```python
from build123d import *

# Parameters (mm, degrees)
SKETCH1_W           = 15.9
SKETCH1_H           = 7.95
BOSS_EXTRUDE1_DEPTH = 3.2
SHELL1_T            = -1.2
SKETCH3_R           = 1.525
SKETCH3_R_2         = 0.5
BOSS_EXTRUDE3_DEPTH = 2
BOSS_EXTRUDE4_DEPTH = 9
SKETCH7_W           = 30
SKETCH7_H           = 30
CUT_EXTRUDE1_DEPTH  = 14.969416324
BOSS_EXTRUDE5_START = -5.621499
SKETCH8_R           = 1.35
BOSS_EXTRUDE5_DEPTH = 5.621499


with BuildPart() as part:
    # Sketch1 → Boss-Extrude1 (new body)
    with BuildSketch(Plane(origin=(0, 0, 0), x_dir=(1, 0, 0), z_dir=(0, 1, 0))):
        Rectangle(SKETCH1_W, SKETCH1_H)
    extrude(amount=BOSS_EXTRUDE1_DEPTH)

    # Shell1
    shell1_openings = [part.faces().sort_by_distance(p)[0] for p in [
        (0, 0, 0),
    ]]
    offset(amount=SHELL1_T, openings=shell1_openings, kind=Kind.INTERSECTION)

    # Sketch3 → Boss-Extrude3 (add)
    with BuildSketch(Plane.XZ.offset(-2)):
        with Locations(Location((0, 0, 0), (0, 0, 270))):
            Circle(SKETCH3_R)
        with Locations(Location((0, 0, 0), (0, 0, 270))):
            Circle(SKETCH3_R_2, mode=Mode.SUBTRACT)
    extrude(amount=BOSS_EXTRUDE3_DEPTH)

    # Sketch4 → Boss-Extrude4 (add)
    with BuildSketch(Plane(origin=(0, 3.2, 0), x_dir=(1, 0, 0), z_dir=(0, 1, 0))):
        with BuildLine():
            Line((-3.9, 3.975), (-3.9, 2.475))
            Line((-3.9, 2.475), (-2.598076211, 2.475))
            ThreePointArc((-2.598076211, 2.475), (0, 0.975), (2.598076211, 2.475))
            Line((2.598076211, 2.475), (3.9, 2.475))
            Line((3.9, 2.475), (3.9, 3.975))
            Line((3.9, 3.975), (-3.9, 3.975))
        make_face()
    extrude(amount=BOSS_EXTRUDE4_DEPTH)

    # Sketch7 → Cut-Extrude1 (cut, through all)
    with BuildSketch(Plane(origin=(0, 4.863093078, 4.863093078), x_dir=(1, 0, 0), z_dir=(0, 0.7071067811865475, 0.7071067811865477))):
        Rectangle(SKETCH7_W, SKETCH7_H)
    extrude(amount=CUT_EXTRUDE1_DEPTH, mode=Mode.SUBTRACT)

    # Sketch8 → Boss-Extrude5 (add)
    with BuildSketch(Plane(origin=(0, 8.0875, 8.0875), x_dir=(1, 0, 0), z_dir=(0, 0.7071067811865475, 0.7071067811865477)).offset(BOSS_EXTRUDE5_START)):
        with Locations(Location((0, 10.087452186, 0), (0, 0, 270))):
            Circle(SKETCH8_R)
    extrude(amount=BOSS_EXTRUDE5_DEPTH)


solid = part.part
```
Build history of the part. All positions in model axes, mm. A direction names the side the tool comes from. Round coordinates to 2 decimals unless told otherwise and drop trailing zeros. Write each loop counter-clockwise with the first axis right and the second up, starting at its lowest first coordinate (ties: lowest second). Pieces come first, ordered by that corner, then holes. Notation, with made-up numbers: (-9, -20.5) - (17, -20.5) arc R22 ccw to (17, 4.5) - close; hole circle Ø9 at (40.5, -8.5). An arc over 180 degrees is marked (long way). Write each question's results on one line, items separated by ' | '. Start each with the question number.
Item 1: Mould opens along Z. For faces 5 (the face through (0, 2, 3.975)), 6 (the face through (3.9, 8, -3)), 7 (the face through (-6.75, 1, 0)) say: pulls with the +Z half, pulls with the -Z half, needs draft (parallel to the pull), parting line crosses it, or undercut.
Item 2: Wall check: L1, parallel to X at y = 0.75, z = 0 (3 decimals); L2, parallel to Z at x = -6.25, y = 1.75 (3 decimals); L3, parallel to Y at x = 4.75, z = 1. Give the ranges that are in metal, low to high. Write a range as [from, to].
Item 3: Saw through at B-B (y = 5.5). Write the cut outline in (x, z) (3 decimals).
Item 4: Saw through at C-C (x = 2.25). Write the cut outline in (y, z) (3 decimals), and give its area (3 significant figures).
Item 5: Saw through at D-D (x = -0.75). Write the cut outline in (y, z) (3 decimals), and give its area (3 significant figures).
Item 6: Saw through at A-A (x = -5.75). Write the cut outline in (y, z) (3 decimals).
Item 7: Which spindle directions (+Z, -Z, +X, -X, +Y, -Y) get a long thin tool onto all of the face, cutting with end or side? Do faces 1 (the face through (3, 8, -2.475)), 2 (the face through (0, 5, -3.975)), 3 (the face through (-0.93, 1.01, 1.21)), 4 (the face through (-3.9, 8, -3)). Say none if no direction does.
Item 8: Drop flat-ended pins along their axis: P1, Ø1.7, axis at x = -3, z = -3, coming from the +Y side; P2, Ø4, axis at x = -6.5, y = 3.5, coming from the +Z side (3 decimals); P3, Ø1.2, axis at x = 1.5, z = -3.5, coming from the +Y side; P4, Ø1.2, axis at y = 9.5, z = -3, coming from the +X side. Give the stop position or say it passes through.
Results are:
1) face 5: pulls with the +Z half | face 6: needs draft | face 7: undercut
2) L1: x = [-7.95, -6.75], [-1.525, -0.5], [0.5, 1.525], [6.75, 7.95] | L2: z = [-3.975, -2.775], [2.775, 3.975] | L3: y = [2, 3.2]
3) outline: (-3.9, -3.975) - (3.9, -3.975) - (3.9, -2.475) - (2.598, -2.475) arc R3 ccw to (-2.598, -2.475) - (-3.9, -2.475) - close
4) outline: (0, -3.975) - (12.2, -3.975) - (12.2, -2.474) - (11.717, -1.991) - (3.2, -1.991) - (3.2, 3.975) - (0, 3.975) - (0, 2.775) - (2, 2.775) - (2, -2.775) - (0, -2.775) - close | area: 32.1 mm²
5) outline: (0, -3.975) - (12.2, -3.975) - (12.2, -3.653) - (16.014, 0.161) - (14.427, 1.748) - (11.202, -1.476) - (10.796, -1.07) - (3.2, -1.07) - (3.2, 3.975) - (0, 3.975) - (0, 2.775) - (2, 2.775) - (2, 1.328) - (0, 1.328) - (0, -1.328) - (2, -1.328) - (2, -2.775) - (0, -2.775) - close | area: 55.4 mm²
6) outline: (0, -3.975) - (3.2, -3.975) - (3.2, 3.975) - (0, 3.975) - (0, 2.775) - (2, 2.775) - (2, -2.775) - (0, -2.775) - close
7) face 1: +Z, +X, +Y | face 2: -Z, +X, -X, +Y, -Y | face 3: -Y | face 4: +Z, -Z, -X, +Y
8) P1: stops at y = 12.2 | P2: stops at z = 3.975 | P3: stops at y = 12.38 | P4: stops at x = 3.9
